The model under review builds one solid part; all positions refer to its coordinate system, in mm. A direction names the side the tool comes from. Coordinates: 2 decimals unless noted, no trailing zeros. Loops run counter-clockwise (first coordinate to the right, second up) from the corner with the lowest first, then second, coordinate; pieces in that order, holes last. Notation, with made-up numbers: (10.5, 18.5) - (67.5, 18.5) arc R24 cw to (67.5, 51.5) - close; hole circle Ø8 at (53, 50.25). An arc over 180 degrees is marked (long way). One line per item, written item: value. Start each with the question number.
1. To check wall thickness, follow line 1 (Y direction, x = 0, z = 3.25); line 2 (Z direction, x = 37, y = -8.5); line 3 (Y direction, x = 0, z = 5.75). State the ranges of each line that lie inside material, in increasing order.
2. Mouldability with a two-part tool opening along Y and no side actions: class faces 3 (the face through (40.06, 12.62, 2.46)), 4 (the face through (4, 0, 7)), 5 (the face through (28, 0, 10)) as +Y half, -Y half, draft (parallel to the pull), parting line (faces both ways), or undercut.
3. We need section A-A, the plane y = 0. Give the boundary of the cut face in (x, z), then the cut area to 3 significant figures.
4. We need section C-C, the plane z = 2.75. Give the boundary of the cut face in (x, y).
5. We need section B-B, the plane x = 0. Give the boundary of the cut face in (y, z), then the cut area to 3 significant figures.
6. Insertion check: P1, Ø3, axis at x = 20.5, z = 6, coming from the -Y side; P2, Ø1, axis at x = 26.5, z = 8, coming from the -Y side; P3, Ø3, axis at x = -2.5, z = 7.5, coming from the +Y side; P4, Ø12, axis at x = -10.5, y = 19, coming from the -Z side. Each pin has a flat end and moves straight along its axis. Give the tip position at first contact, or say it passes through.
7. For faces 1 (the face through (-29.987, 0.88, 7.465)), 2 (the face through (-3, 0, 5)), list the 3-axis set-ups (+Z, -Z, +X, -X, +Y, -Y) from which the entire face can be reached by the end or side of a thin tool; tool diameter is ignored.
8. We need section D-D, the plane x = -17. Give the boundary of the cut face in (y, z).
from build123d import *

# Parameters (mm, degrees)
SKETCH_R     = 42
PAD_DEPTH    = 5
SKETCH001_R  = 3
PAD001_DEPTH = 5
PAD002_DEPTH = 5
SKETCH003_R  = 3
POCKET_DEPTH = 10


with BuildPart() as part:
    # Sketch → Pad (new body)
    with BuildSketch(Plane.XY):
        Circle(SKETCH_R)
    extrude(amount=PAD_DEPTH)

    # Sketch001 → Pad001 (new body)
    with BuildSketch(Plane.XY.offset(5)):
        with Locations((28, 0)):
            Circle(SKETCH001_R)
    extrude(amount=PAD001_DEPTH)

    # Sketch002 → Pad002 (new body)
    with BuildSketch(Plane.XY.offset(5)):
        with BuildLine():
            ThreePointArc((15.05, 25.95183), (4, 0), (15.05, -25.95183))
            ThreePointArc((15.05, 25.95183), (-30, 0), (15.05, -25.95183))
        make_face()
    extrude(amount=PAD002_DEPTH)

    # Sketch003 → Pocket (cut)
    with BuildSketch(Plane(origin=(0, 0, 0), x_dir=(1, 0, 0), z_dir=(0, 0, -1))):
        Circle(SKETCH003_R)
    extrude(amount=-POCKET_DEPTH, mode=Mode.SUBTRACT)


solid = part.part
Findings below:
1. line 1: -42 to -3, 3 to 42
1. line 2: 0 to 5
1. line 3: -30 to -3, 3 to 30
2. face 3: parting line
2. face 4: undercut
2. face 5: draft
3. outline: (-42, 0) - (-3, 0) - (-3, 10) - (-30, 10) - (-30, 5) - (-42, 5) - close; (3, 0) - (42, 0) - (42, 5) - (31, 5) - (31, 10) - (25, 10) - (25, 5) - (4, 5) - (4, 10) - (3, 10) - close
3. area: 560 mm2
4. outline: circle Ø84 at (0, 0); hole circle Ø6 at (0, 0)
5. outline: (-42, 0) - (-3, 0) - (-3, 10) - (-30, 10) - (-30, 5) - (-42, 5) - close; (3, 0) - (42, 0) - (42, 5) - (30, 5) - (30, 10) - (3, 10) - close
5. area: 660 mm2
6. P1: y = -37.26
6. P2: y = -2.83
6. P3: y = 29.98
6. P4: z = 0
7. face 1: +Z
7. face 2: +Z, -Z
8. outline: (-38.41, 0) - (38.41, 0) - (38.41, 5) - (24.72, 5) - (24.72, 10) - (-24.72, 10) - (-24.72, 5) - (-38.41, 5) - close
